```python
from build123d import *

# Parameters (mm, degrees)
BASE_EXTRUDE_DEPTH                 = 5
CUTAWAY_FOR_CLAMP_PLATE_WIRE_DEPTH = 11
HOLES_TO_PITCH_PLATE_REACH         = 22
SKETCH4_R                          = 2.15265
SKETCH5_R                          = 2.05
EXTRUDE1_DEPTH                     = 4
SKETCH6_R                          = 0.75
EXTRUDE2_DEPTH                     = 2
SKETCH8_W                          = 18.476012794
SKETCH8_H                          = 10
SKETCH8_R                          = 2.15265
EXTRUDE3_DEPTH                     = 5.102995
SKETCH7_R                          = 2.05
CUT_EXTRUDE1_DEPTH                 = 25.066935872
CUT_EXTRUDE3_REACH                 = 32.496
SKETCH12_W                         = 1.1
SKETCH12_H                         = 6
F_8_32_TAPPED_HOLE1_D              = 3.4544
F_8_32_TAPPED_HOLE1_DEPTH          = 6.858
F_8_32_TAPPED_HOLE1_TIP            = 1.037806461


with BuildPart() as part:
    # Sketch1 → Base-Extrude (new body, symmetric)
    with BuildSketch(Plane.XY):
        Polygon((-7.703086391, 2.967740731), (0, 0), (7.703086391, -2.967740731), (1.037503031, -20.268970563), (-25.460082654, -20.268970563), (-25.460082654, -0.268970563), (-8.950082654, -0.268970563), align=None)
    extrude(amount=BASE_EXTRUDE_DEPTH, both=True)

    # Sketch2 → Cutaway for Clamp Plate & Wire (cut, through all)
    with BuildSketch(Plane.XY.offset(5)):
        Polygon((-7.703086391, 2.967740731), (7.703086391, -2.967740731), (1.037503031, -20.268970563), (-8.607332328, -20.268970563), (-2.133223778, -3.464733945), (-9.141119453, -0.764826872), align=None)
    extrude(amount=-CUTAWAY_FOR_CLAMP_PLATE_WIRE_DEPTH, mode=Mode.SUBTRACT)

    # Sketch4 → Holes to Pitch Plate (cut, up to next)
    with BuildSketch(Plane(origin=(0, -0.268970563, 0), x_dir=(-1, 0, 0), z_dir=(0, 1, 0)), mode=Mode.PRIVATE) as holes_to_pitch_plate_sk1:
        with Locations((21.332582654, 0)):
            Circle(SKETCH4_R)
    holes_to_pitch_plate_tool1 = extrude(holes_to_pitch_plate_sk1.sketch, amount=-HOLES_TO_PITCH_PLATE_REACH, mode=Mode.PRIVATE) & part.part
    add(holes_to_pitch_plate_tool1.solids().sort_by_distance((-21.332583, -0.268971, 0))[0], mode=Mode.SUBTRACT)
    # Sketch4 → Holes to Pitch Plate (cut, up to next)
    with BuildSketch(Plane(origin=(0, -0.268970563, 0), x_dir=(-1, 0, 0), z_dir=(0, 1, 0)), mode=Mode.PRIVATE) as holes_to_pitch_plate_sk2:
        with Locations(Location((13.077582654, 0, 0), (0, 0, 90))):  # turned: the seam where the file's is
            Circle(SKETCH4_R)
    holes_to_pitch_plate_tool2 = extrude(holes_to_pitch_plate_sk2.sketch, amount=-HOLES_TO_PITCH_PLATE_REACH, mode=Mode.PRIVATE) & part.part
    add(holes_to_pitch_plate_tool2.solids().sort_by_distance((-13.077583, -0.268971, 0))[0], mode=Mode.SUBTRACT)

    # Sketch5 → Extrude1 (add)
    with BuildSketch(Plane(origin=(-1.438033062, -3.732567603, 0), x_dir=(-0.933141901, 0.359508265, 0), z_dir=(0.359508265, 0.933141901, 0))):
        Polygon((8.255, 5), (0, 5), (-5, 5), (-5, -5), (0, -5), (8.255, -5), align=None)
        with Locations(Location((0, 0, 0), (0, 0, 291.310049103))):  # turned: the seam where the file's is
            Circle(SKETCH5_R, mode=Mode.SUBTRACT)
    extrude(amount=EXTRUDE1_DEPTH)

    # Sketch6 → Extrude2 (add)
    with BuildSketch(Plane(origin=(0, 0, 0), x_dir=(-0.933141901, 0.359508265, 0), z_dir=(0.359508265, 0.933141901, 0))):
        Polygon((0, 5), (8.255, 5), (8.255, -5), (0, -5), (-5, -5), (-5, 5), align=None)
        Circle(SKETCH6_R, mode=Mode.SUBTRACT)
    extrude(amount=EXTRUDE2_DEPTH)

    # Sketch8 → Extrude3 (add)
    with BuildSketch(Plane(origin=(0, -0.268970563, 0), x_dir=(-1, 0, 0), z_dir=(0, 1, 0))):
        with Locations((16.222076257, 0)):
            Rectangle(SKETCH8_W, SKETCH8_H)
        with Locations(Location((21.332582654, 0, 0), (0, 0, 90))):  # turned: the seam where the file's is
            Circle(SKETCH8_R, mode=Mode.SUBTRACT)
        with Locations(Location((13.077582654, 0, 0), (0, 0, 90))):  # turned: the seam where the file's is
            Circle(SKETCH8_R, mode=Mode.SUBTRACT)
    extrude(amount=EXTRUDE3_DEPTH)

    # Sketch7 → Cut-Extrude1 (cut, through all)
    with BuildSketch(Plane(origin=(-1.438033062, -3.732567603, 0), x_dir=(0.933141901, -0.359508265, 0), z_dir=(-0.359508265, -0.933141901, 0))):
        with Locations(Location((0, 0, 0), (0, 0, 248.689950897))):  # turned: the seam where the file's is
            Circle(SKETCH7_R)
    extrude(amount=CUT_EXTRUDE1_DEPTH, mode=Mode.SUBTRACT)

    # Sketch12 → Cut-Extrude3 (cut, up to next)
    with BuildSketch(Plane(origin=(4.665709504, -1.797541327, 0), x_dir=(0, 0, -1), z_dir=(0.933141901, -0.359508265, 0)), mode=Mode.PRIVATE) as cut_extrude3_sk1:
        with Locations((0, -1)):
            Rectangle(SKETCH12_W, SKETCH12_H)
    cut_extrude3_tool1 = extrude(cut_extrude3_sk1.sketch, amount=-CUT_EXTRUDE3_REACH, mode=Mode.PRIVATE) & part.part
    add(cut_extrude3_tool1.solids().sort_by_distance((4.306201, -2.730683, 0))[0], mode=Mode.SUBTRACT)

    # #8-32 Tapped Hole1
    with Locations(Plane(origin=(-0.695190716, 0.267833658, 0), x_dir=(0, 0, -1), z_dir=(0.933141901, -0.359508265, 0))):
        with Locations((-0.041026912, -7.429)):
            Hole(F_8_32_TAPPED_HOLE1_D / 2, depth=F_8_32_TAPPED_HOLE1_DEPTH)
            with Locations((0, 0, -(F_8_32_TAPPED_HOLE1_DEPTH + F_8_32_TAPPED_HOLE1_TIP / 2))):  # 118° drill point
                Cone(0, F_8_32_TAPPED_HOLE1_D / 2, F_8_32_TAPPED_HOLE1_TIP, mode=Mode.SUBTRACT)


solid = part.part
```
Work out the finished part from the listing and answer in its coordinate system (mm). A direction names the side the tool comes from. Give positions to 0.01 mm unless a question says otherwise; leave off trailing zeros. Order: outer loops, then holes, each group sorted by start corner. A loop starts at its lowest first (then second) coordinate and runs counter-clockwise, first axis right, second up.
1. This flat-tipped pin is pushed along its axis until it touches: P1, Ø1.5, axis at y = 0.5, z = -3.5, coming from the +X side. Where does it stop, or does it pass through?
Result sheet:
P1: stops at x = 5.38
2. For faces 1 (the flat face through (0.58, -4.51, -2.74)), 2 (the flat face through (3, -2, 0.55)), 3 (the flat face through (-13, -8, -5)), 4 (the flat face through (-0.886, 2.485, 0.07)), 5 (the flat face through (-0.896, 0.345, 0.029)), determine the directions among +Z, -Z, +X, -X, +Y, -Y from which every point of the face is accessible in a straight line to the end or side of a thin tool.
Result sheet:
face 1: +Z, -Z, -Y
face 2: +X, +Y, -Y
face 3: -Z, +X, -X, +Y, -Y
face 4: +Z, -Z, +X, +Y
face 5: none
3. Section A-A, the plane x = -22 is taken. Determine the outline of the cut face in (y, z), and give its area (3 significant figures).
Result sheet:
outline: (-20.27, -5) - (4.83, -5) - (4.83, -2.05) - (-20.27, -2.05) - close; (-20.27, 2.05) - (4.83, 2.05) - (4.83, 5) - (-20.27, 5) - close
area: 148 mm2
4. Section B-B, the plane z = 3.75 is taken. Determine the outline of the cut face in (x, y), and give its area (3 significant figures).
Result sheet:
outline: (-25.46, -20.27) - (-8.61, -20.27) - (-2.13, -3.46) - (3.23, -5.53) - (5.38, 0.07) - (-6.98, 4.83) - (-25.46, 4.83) - close
area: 568 mm2
5. The mould has two halves that part along Z. Classify faces 6 (the flat face through (3, -2, -0.55)), 7 (the flat face through (-16, 4.834, 0)), 8 (the flat face through (-13, -5, 5)): released by +Z, released by -Z, zero draft, split by the parting line, or undercut.
Result sheet:
face 6: undercut
face 7: zero draft
face 8: released by +Z
6. Straight lines are drawn through the part: L1, parallel to Z at x = -20, y = -13.25; L2, parallel to X at y = -10.25, z = 0; L3, parallel to X at y = -12.75, z = 0. For each, find the intervals that lie inside material, in ascending order.
Result sheet:
L1: z = -5 to -1.69, 1.69 to 5
L2: x = -25.46 to -23.49, -19.18 to -15.23, -10.92 to -6.15
L3: x = -25.46 to -23.49, -19.18 to -15.23, -10.92 to -7.11
